Model file for the job. Use its own axes, mm. A direction names the side the tool comes from. Coordinates: 2 decimals unless noted, no trailing zeros. Loops run counter-clockwise (first coordinate to the right, second up) from the corner with the lowest first, then second, coordinate; pieces in that order, holes last. Notation, with made-up numbers: (57, -11) - (66, -11) arc R26 cw to (66, 3) - close; hole circle Ø3 at (38.25, 78.5). An arc over 180 degrees is marked (long way). Write each question's results on one line, items separated by ' | '. Start each with the question number.
```python
from build123d import *

# Parameters (mm, degrees)
F0_R     = 16.5
F1_DEPTH = 8
F2_R     = 1.1
F3_DEPTH = 2.5
F4_R     = 1
F5_DEPTH = 2.5


with BuildPart() as f1:
    # F0 (on Top) → F1 (new body)
    with BuildSketch(Plane.XY):
        Circle(F0_R)
    extrude(amount=F1_DEPTH)

    # F2 (on face) → F3 (cut)
    with BuildSketch(Plane(origin=(0, 0, 0), x_dir=(1, 0, 0), z_dir=(0, 0, -1))):
        with Locations((0, 15.1)):
            Circle(F2_R)
        with Locations((15, 0.1)):
            Circle(F2_R)
        with Locations((0, -14.9)):
            Circle(F2_R)
    extrude(amount=-F3_DEPTH, mode=Mode.SUBTRACT)

    # F4 (on face) → F5 (join)
    with BuildSketch(Plane.XY.offset(8)):
        with Locations((0, 15)):
            Circle(F4_R)
        with Locations((15, 0)):
            Circle(F4_R)
        with Locations((0, -15)):
            Circle(F4_R)
    extrude(amount=F5_DEPTH)


solid = f1.part
```
Q1. Which spindle directions (+Z, -Z, +X, -X, +Y, -Y) get a long thin tool onto all of the face, cutting with end or side? Do faces 1 (the cylindrical face through (-0.14, -16.19, 1.23)), 2 (the flat face through (15, 0, 10.5)), 3 (the cylindrical face through (0, -16, 9)). Say none if no direction does.
Q2. Pin check, flat tips, straight feed: pin 1 (5 mm diameter, centred on x = -11.5, z = 5, fed in from -Y); pin 2 (2 mm diameter, centred on y = -1.5, z = 2.5, fed in from +X); pin 3 (10 mm diameter, centred on x = -11, y = 1, fed in from +Z). Stop position of each tip, or through.
Q3. Drill centre lines: L1, parallel to Y at x = 0, z = 1.5; L2, parallel to Z at x = 6.5, y = -6; L3, parallel to Y at x = 1, z = 2. Where is each one in solid material? Low to high. Write a range as from..to.
Q4. Mould opens along X. For faces 4 (the cylindrical face through (0, 14, 9)), 5 (the cylindrical face through (13.9, -0.1, 1.2)), 6 (the flat face through (0, 15, 2.5)), 7 (the flat face through (0, 15, 10.5)) say: +X half, -X half, draft (parallel to the pull), parting line (faces both ways), or undercut.
Q5. Cut at A-A (x = 15). List the corners of the cut face in (y, z).
Q6. Cut at C-C (y = -12.5). List the corners of the cut face in (x, z), and give its area (3 significant figures).
Q7. Cut at D-D (x = -11). List the corners of the cut face in (y, z), and give its area (3 significant figures).
Q8. Cut at B-B (z = 3.75). List the corners of the cut face in (x, y).
Check result:
1) face 1: -Z | face 2: +Z, +X, -X, +Y, -Y | face 3: +Z
2) pin 1: y = -13.83 | pin 2: x = 16.49 | pin 3: z = 8
3) L1: -16.5..-16.2, -14..13.8, 16..16.5 | L2: 0..8 | L3: -16.47..-15.56, -14.64..14.44, 15.36..16.47
4) face 4: parting line | face 5: undercut | face 6: undercut | face 7: draft
5) outline: (-6.87, 0) - (-1.2, 0) - (-1.2, 2.5) - (1, 2.5) - (1, 0) - (6.87, 0) - (6.87, 8) - (1, 8) - (1, 10.5) - (-1, 10.5) - (-1, 8) - (-6.87, 8) - close
6) outline: (-10.77, 0) - (10.77, 0) - (10.77, 8) - (-10.77, 8) - close | area: 172 mm²
7) outline: (-12.3, 0) - (12.3, 0) - (12.3, 8) - (-12.3, 8) - close | area: 197 mm²
8) outline: circle Ø33 at (0, 0)
